Part model, mm, in its own coordinate system. Round coordinates to 2 decimals unless told otherwise and drop trailing zeros. Write each loop counter-clockwise with the first axis right and the second up, starting at its lowest first coordinate (ties: lowest second). Pieces come first, ordered by that corner, then holes. Notation, with made-up numbers: M -10.5,-22 L 8.5,-22 A24 ccw 8.5,15 Z; hole C -3.75,61 d5. An arc over 180 degrees is marked long. One line per question, with ' | ' between items. Start each with the question number.
1) Wall check: probe 1 along X at (y, z) = (2, -8); probe 2 along Z at (x, y) = (12, 2); probe 3 along X at (y, z) = (4.5, 8). Give the ranges that are in metal, low to high. Write a range as [from, to].
2) Saw through at A-A (x = 0). List the corners of the cut face in (y, z), plus the area to 3 significant figures.
3) Saw through at B-B (z = -11.5). List the corners of the cut face in (x, y), plus the area to 3 significant figures.
4) Saw through at D-D (x = 8.5). List the corners of the cut face in (y, z).
5) Saw through at C-C (z = -8). List the corners of the cut face in (x, y), plus the area to 3 significant figures.
6) Mould opens along Z. For faces 1 (the face through (-12.13, 3.22, 4.72)), 2 (the face through (-14.148, 3.219, 9.947)), 3 (the face through (0, 0, -10)) say: pulls with the +Z half, pulls with the -Z half, needs draft (parallel to the pull), parting line crosses it, or undercut.
```python
from build123d import *

# Parameters (mm, degrees)
BOSS_EXTRUDE1_DEPTH              = 6.35
F_2_2_2_2_DIAMETER_HOLE1_D       = 2.2
F_2_2_2_2_DIAMETER_HOLE1_DEPTH   = 6.35
F_2_2_2_2_DIAMETER_HOLE2_D       = 2.2
F_2_2_2_2_DIAMETER_HOLE2_DEPTH   = 6.35
F_2_2_2_2_DIAMETER_HOLE3_D       = 2.2
F_2_2_2_2_DIAMETER_HOLE3_DEPTH   = 6.35
F_2_2_2_2_DIAMETER_HOLE4_D       = 2.2
F_2_2_2_2_DIAMETER_HOLE4_DEPTH   = 6.35
F_18_5_18_5_DIAMETER_HOLE1_D     = 18.5
F_18_5_18_5_DIAMETER_HOLE1_DEPTH = 6.35
M3_TAPPED_HOLE1_D                = 2.5
M3_TAPPED_HOLE2_D                = 2.5
M3_TAPPED_HOLE3_D                = 2.5
M3_TAPPED_HOLE4_D                = 2.5


with BuildPart() as part:
    # Sketch1 → Boss-Extrude1 (new body)
    with BuildSketch(Plane(origin=(0, 6.35, 0), x_dir=(1, 0, 0), z_dir=(0, 1, 0))):
        with BuildLine():
            Line((15.288980095, -7.15), (15.288980095, 14))
            Line((15.288980095, 14), (-15.289019905, 14))
            Line((-15.289019905, 14), (-15.289019905, -7.15))
            ThreePointArc((-15.289019905, -7.15), (-14.11744703, -9.978427125), (-11.289019905, -11.15))
            Line((-11.289019905, -11.15), (11.288980095, -11.15))
            ThreePointArc((11.288980095, -11.15), (14.11740722, -9.978427125), (15.288980095, -7.15))
        make_face()
    extrude(amount=-BOSS_EXTRUDE1_DEPTH)

    # Ø2.2 (2.2) Diameter Hole1
    with Locations(Plane(origin=(0, 0, 0), x_dir=(-1, 0, 0), z_dir=(0, -1, 0))):
        with Locations((-7.999980095, -8)):
            Hole(F_2_2_2_2_DIAMETER_HOLE1_D / 2, depth=F_2_2_2_2_DIAMETER_HOLE1_DEPTH)

    # Ø2.2 (2.2) Diameter Hole2
    with Locations(Plane(origin=(0, 0, 0), x_dir=(-1, 0, 0), z_dir=(0, -1, 0))):
        with Locations((8.000019905, 8)):
            Hole(F_2_2_2_2_DIAMETER_HOLE2_D / 2, depth=F_2_2_2_2_DIAMETER_HOLE2_DEPTH)

    # Ø2.2 (2.2) Diameter Hole3
    with Locations(Plane(origin=(0, 0, 0), x_dir=(-1, 0, 0), z_dir=(0, -1, 0))):
        with Locations((-7.999980095, 8)):
            Hole(F_2_2_2_2_DIAMETER_HOLE3_D / 2, depth=F_2_2_2_2_DIAMETER_HOLE3_DEPTH)

    # Ø2.2 (2.2) Diameter Hole4
    with Locations(Plane(origin=(0, 6.35, 0), x_dir=(1, 0, 0), z_dir=(0, 1, 0))):
        with Locations((-8.000019905, -8)):
            Hole(F_2_2_2_2_DIAMETER_HOLE4_D / 2, depth=F_2_2_2_2_DIAMETER_HOLE4_DEPTH)

    # Ø18.5 (18.5) Diameter Hole1
    with Locations(Plane(origin=(0, 0, 0), x_dir=(-1, 0, 0), z_dir=(0, -1, 0))):
        with Locations((0, 0)):
            Hole(F_18_5_18_5_DIAMETER_HOLE1_D / 2, depth=F_18_5_18_5_DIAMETER_HOLE1_DEPTH)

    # M3 Tapped Hole1 (through all)
    with Locations(Plane(origin=(0, 0, 0), x_dir=(-1, 0, 0), z_dir=(0, -1, 0))):
        with Locations((11.858637076, 11.5)):
            Hole(M3_TAPPED_HOLE1_D / 2)

    # M3 Tapped Hole2 (through all)
    with Locations(Plane(origin=(0, 0, 0), x_dir=(-1, 0, 0), z_dir=(0, -1, 0))):
        with Locations((11.85956559, -3.500033723)):
            Hole(M3_TAPPED_HOLE2_D / 2)

    # M3 Tapped Hole3 (through all)
    with Locations(Plane(origin=(0, 0, 0), x_dir=(-1, 0, 0), z_dir=(0, -1, 0))):
        with Locations((-11.858647005, 11.5)):
            Hole(M3_TAPPED_HOLE3_D / 2)

    # M3 Tapped Hole4 (through all)
    with Locations(Plane(origin=(0, 0, 0), x_dir=(-1, 0, 0), z_dir=(0, -1, 0))):
        with Locations((-11.859575542, -3.5)):
            Hole(M3_TAPPED_HOLE4_D / 2)


solid = part.part
```
Answer key:
1) probe 1: x = [-15.29, -9.1], [-6.9, -4.64], [4.64, 6.9], [9.1, 15.29] | probe 2: z = [-14, -12.74], [-10.26, 2.26], [4.74, 11.09] | probe 3: x = [-15.2, -9.1], [-6.9, -4.64], [4.64, 6.9], [9.1, 15.2]
2) outline: M 0,-14 L 6.35,-14 L 6.35,-9.25 L 0,-9.25 Z; M 0,9.25 L 6.35,9.25 L 6.35,11.15 L 0,11.15 Z | area: 42.2 mm2
3) outline: M -15.29,0 L -13.11,0 L -13.11,6.35 L -15.29,6.35 Z; M -10.61,0 L 10.61,0 L 10.61,6.35 L -10.61,6.35 Z; M 13.11,0 L 15.29,0 L 15.29,6.35 L 13.11,6.35 Z | area: 162 mm2
4) outline: M 0,-14 L 6.35,-14 L 6.35,-8.98 L 0,-8.98 Z; M 0,-7.02 L 6.35,-7.02 L 6.35,-3.65 L 0,-3.65 Z; M 0,3.65 L 6.35,3.65 L 6.35,7.02 L 0,7.02 Z; M 0,8.98 L 6.35,8.98 L 6.35,11.15 L 0,11.15 Z
5) outline: M -15.29,0 L -9.1,0 L -9.1,6.35 L -15.29,6.35 Z; M -6.9,0 L -4.64,0 L -4.64,6.35 L -6.9,6.35 Z; M 4.64,0 L 6.9,0 L 6.9,6.35 L 4.64,6.35 Z; M 9.1,0 L 15.29,0 L 15.29,6.35 L 9.1,6.35 Z | area: 107 mm2
6) face 1: undercut | face 2: pulls with the +Z half | face 3: needs draft
